```python
from build123d import *

# Parameters (mm, degrees)
ESQUISSE1_W        = 60.213993324
ESQUISSE1_H        = 46
BOSS_EXTRU_1_DEPTH = 5
ESQUISSE2_W        = 8
ESQUISSE2_H        = 46
ESQUISSE2_W_2      = 15.12622911
BOSS_EXTRU_2_DEPTH = 6
ESQUISSE8_R        = 11
BOSS_EXTRU_4_DEPTH = 8
ESQUISSE10_W       = 12
ESQUISSE10_H       = 46
BOSS_EXTRU_5_DEPTH = 15.12622911


with BuildPart() as part:
    # Esquisse1 → Boss.-Extru.1 (new body)
    with BuildSketch(Plane.XY):
        with Locations((-16.106996662, 0)):
            Rectangle(ESQUISSE1_W, ESQUISSE1_H)
    extrude(amount=BOSS_EXTRU_1_DEPTH)

    # Esquisse2 → Boss.-Extru.2 (add)
    with BuildSketch(Plane.XY.offset(5)):
        with Locations((9, 0)):
            Rectangle(ESQUISSE2_W, ESQUISSE2_H)
        with Locations((-16.60101476, 0)):
            Rectangle(ESQUISSE2_W_2, ESQUISSE2_H)
    extrude(amount=BOSS_EXTRU_2_DEPTH)

    # Esquisse8 → Boss.-Extru.4 (add)
    with BuildSketch(Plane.ZY.offset(-5)):
        with BuildLine():
            Line((33, -23), (11, -23))
            Line((11, -23), (11, 23))
            Line((11, 23), (33, 23))
            ThreePointArc((33, 23), (56, 0), (33, -23))
        make_face()
        with Locations((33, 0)):
            Circle(ESQUISSE8_R, mode=Mode.SUBTRACT)
    extrude(amount=-BOSS_EXTRU_4_DEPTH)

    # Esquisse10 → Boss.-Extru.5 (add)
    with BuildSketch(Plane.ZY.offset(24.164129315)):
        with Locations((17, 0)):
            Rectangle(ESQUISSE10_W, ESQUISSE10_H)
    extrude(amount=-BOSS_EXTRU_5_DEPTH)


solid = part.part
```
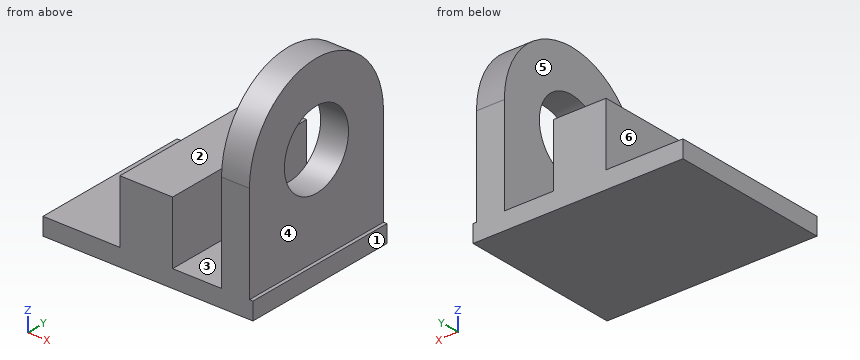
Geometry check sheet. Reference: the model listing, model coordinates, mm. Face numbers are marked on the shaded views. A direction names the side the tool comes from. Give positions to 0.01 mm unless a question says otherwise; leave off trailing zeros. Loops run counter-clockwise (first coordinate to the right, second up) from the corner with the lowest first, then second, coordinate; pieces in that order, holes last. Notation, with made-up numbers: M -14,-5 L 10,-5 A31 ccw 10,23 Z; hole C 45,5 d11. An arc over 180 degrees is marked long. Answer as CSV lines item,"result".
Item 1: Material ranges on line 1 (X direction, y = -14, z = 15); line 2 (Y direction, x = 7, z = 33); line 3 (Z direction, x = -41, y = -6), recorded low to high.
Values:
line 1,"x = -24.16 to -9.04, 5 to 13"
line 2,"y = -23 to -11, 11 to 23"
line 3,"z = 0 to 5"
Item 2: Cross-section at B-B on y = 0. Record the cut outline in (x, z), and give its area (3 significant figures).
Values:
outline,"M -46.21,0 L 14,0 L 14,5 L 13,5 L 13,22 L 5,22 L 5,5 L -9.04,5 L -9.04,23 L -24.16,23 L -24.16,5 L -46.21,5 Z; M 5,44 L 13,44 L 13,56 L 5,56 Z"
area,"805 mm²"
Item 3: Cross-section at A-A on z = 18.5. Record the cut outline in (x, y), and give its area (3 significant figures).
Values:
outline,"M -24.16,-23 L -9.04,-23 L -9.04,23 L -24.16,23 Z; M 5,-23 L 13,-23 L 13,23 L 5,23 Z"
area,"1,060 mm²"
Item 4: Cross-section at C-C on x = 8.5. Record the cut outline in (y, z).
Values:
outline,"M -23,0 L 23,0 L 23,33 A23 ccw -23,33 Z; hole C 0,33 d22"
Item 5: Release check for a two-part mould opening along X. For the marked faces 4, 5 and 6 record: pulls with the +X half, pulls with the -X half, needs draft (parallel to the pull), parting line crosses it, or undercut.
Values:
face 4,"pulls with the +X half"
face 5,"undercut"
face 6,"pulls with the -X half"
Item 6: Depth check by flat-ended pin: P1, Ø24.5, axis at x = -30, y = 2, coming from the +Z side; P2, Ø3, axis at y = 2.5, z = 7.5, coming from the +X side; P3, Ø3, axis at x = -28.5, y = 17.5, coming from the +Z side. Enter the tip coordinate at first touch or a pass-through.
Values:
P1,"stops at z = 23"
P2,"stops at x = 13"
P3,"stops at z = 5"
Item 7: Cross-section at D-D on y = 12. Record the cut outline in (x, z), and give its area (3 significant figures).
Values:
outline,"M -46.21,0 L 14,0 L 14,5 L 13,5 L 13,52.62 L 5,52.62 L 5,5 L -9.04,5 L -9.04,23 L -24.16,23 L -24.16,5 L -46.21,5 Z"
area,"954 mm²"
Item 8: Access from +Z, -Z, +X, -X, +Y, -Y to the whole of each face (thin tool, end or side, straight path). Record for the marked faces 1, 2 and 3.
Values:
face 1,"+Z, -Z, +X, +Y, -Y"
face 2,"+Z, -X, +Y, -Y"
face 3,"+Z, +Y, -Y"
